Geometry: final body of the model. Coordinates: model frame, mm. A direction names the side the tool comes from. Give positions to 0.01 mm unless a question says otherwise; leave off trailing zeros. Order: outer loops, then holes, each group sorted by start corner. A loop starts at its lowest first (then second) coordinate and runs counter-clockwise, first axis right, second up. Notation, with made-up numbers: (27, 31.5) -> (38, 31.5) arc R24 ccw to (38, 55.5) -> close; hole circle Ø1 at (71, 35). An arc over 180 degrees is marked (long way). Write item = value, one per line.
Autodesk Inventor part; units mm, degrees
ref_plane "YZ Plane" through (0, 0, 0) normal (1, 0, 0) x (0, 1, 0)
ref_plane "XZ Plane" through (0, 0, 0) normal (0, 1, 0) x (-1, 0, 0)
ref_plane "XY Plane" through (0, 0, 0) normal (0, 0, 1) x (1, 0, 0)
sketch "Sketch1" plane through (0, 0, 0) normal (0, 0, 1) x (1, 0, 0)
  circle A0 centre (0, 0) radius 5.75
  circle A1 centre (0, 8) radius 2
  circle A2 centre (8, 0) radius 2
  circle A3 centre (0, -8) radius 2
  circle A4 centre (-8, 0) radius 2
  line L0 (-15, 17.5) -> (15, 17.5)
  line L1 (15, 17.5) -> (15, -17.5)
  line L2 (15, -17.5) -> (-15, -17.5)
  line L3 (-15, -17.5) -> (-15, 17.5)
  line L4 (-15, 17.5) -> (15, -17.5) construction
  line L5 (15, 17.5) -> (-15, -17.5) construction
  dimension "d0" = 11.5
  dimension "d2" = 4
  dimension "d3" = 4
  dimension "d4" = 4
  dimension "d5" = 4
  dimension "d6" = 30
  dimension "d7" = 35
extrude "Extrusion1" add sketch "Sketch1" along normal blind 25
sketch "Sketch2" plane through (-15, -17.5, 0) normal (0, -1, 0) x (1, 0, 0)
  line L0 (0, 0) -> (0, 25)
  line L1 (30, 0) -> (0, 0)
  line L2 (0, 25) -> (30, 0)
  line L3 (-15, 32.5) -> (45, 32.5)
  line L4 (45, 32.5) -> (45, -7.5)
  line L5 (45, -7.5) -> (-15, -7.5)
  line L6 (-15, -7.5) -> (-15, 32.5)
  line L7 (-15, 32.5) -> (45, -7.5) construction
  line L8 (45, 32.5) -> (-15, -7.5) construction
  point P0 (15, 0)
  point P1 (15, 12.5)
  dimension "d10" = 60
  dimension "d11" = 40
extrude "Extrusion2" add sketch "Sketch2" along normal blind 6 contours L0 L2 L1 | L3 L4 L5 L6
sketch "Sketch3" plane through (-15, -23.5, 0) normal (0, -1, 0) x (1, 0, 0)
  line L0 (-15, -7.5) -> (-15, 32.5)
  line L1 (45, 32.5) -> (45, -7.5)
  line L2 (-15, 26) -> (45, 26)
  line L3 (-15, 19) -> (45, 19)
  line L4 (-15, 6) -> (45, 6)
  line L5 (-15, -1) -> (45, -1)
  line L6 (45, 26) -> (45, 19)
  line L7 (45, 6) -> (45, -1)
  line L8 (-15, -1) -> (-15, 6)
  line L9 (-15, 19) -> (-15, 26)
  point P0 (15, 0)
extrude "Extrusion3" add sketch "Sketch3" along normal blind 1.5 contours L0 L4 L1 L5 | L0 L2 L1 L3
sketch "Sketch4" plane through (-15, -25, 0) normal (0, -1, 0) x (1, 0, 0)
  line L0 (-15, 26) -> (45, 26)
  line L1 (45, 26) -> (30, 19)
  line L2 (-15, 19) -> (45, 19)
  line L3 (30, 0) -> (30, 25)
  line L4 (30, 13) -> (5, 13)
  line L5 (5, 0) -> (5, 25)
  line L6 (45, -7.5) -> (-15, -7.5)
  line L7 (15, -7.5) -> (15, 32.5)
  line L8 (45, 32.5) -> (-15, 32.5)
  point P0 (15, 0)
  point P1 (37.5, 22.5)
  point P2 (37.5, 3.5)
  point P3 (-7.5, 22.5)
  point P4 (-7.5, 3.5)
hole "Hole1" at (22.5, -25, 22.5) at (22.5, -25, 3.5) at (-22.5, -25, 22.5) at (-22.5, -25, 3.5) direction (0, 1, 0) diameter 5.5 end through all counterbore diameter 10 counterbore depth 1.5
fillet "Fillet1" radius 2 8 edges at (15, 17.5, 12.5) (0, 17.5, 25) (-15, 17.5, 12.5) (0, 17.5, 0) (-30, -20.5, -7.5) (30, -20.5, -7.5) (30, -20.5, 32.5) (-30, -20.5, 32.5)
properties part number "CarroZ - EixoZ"
1) Section query C-C (x = 22.5). Output: boundary loops of the cut face in (y, z), plus the area to 3 significant figures.
Check sheet entries:
outline = (-23.5, -7.5) -> (-17.5, -7.5) -> (-17.5, 0.75) -> (-23.5, 0.75) -> close; (-23.5, 6.25) -> (-17.5, 6.25) -> (-17.5, 19.75) -> (-23.5, 19.75) -> close; (-23.5, 25.25) -> (-17.5, 25.25) -> (-17.5, 32.5) -> (-23.5, 32.5) -> close
area = 174 mm²
2) First-contact query: P1, Ø10, axis at x = 21.5, y = -16, coming from the +Z side; P2, Ø10, axis at x = -6, y = 3, coming from the -Z side; P3, Ø6.5, axis at x = 22.5, z = 3.5, coming from the -Y side; P4, Ø5, axis at x = 22.5, z = 22.5, coming from the -Y side. Flat tips, straight axial feed; report the tip coordinate or a pass-through.
Check sheet entries:
P1 = 32.5
P2 = 0
P3 = -23.5
P4 = through
3) Line query: line 1 (X direction, y = -19.1, z = 22.5); line 2 (Z direction, x = -22.5, y = -21.45); line 3 (Y direction, x = 0, z = 15.5). Output: solid intervals per line, ascending. Write a range as from..to.
Check sheet entries:
line_1 = -30..-25.25, -19.75..19.75, 25.25..30
line_2 = -7.5..0.75, 6.25..19.75, 25.25..32.5
line_3 = -23.5..-10, -6..-5.75, 5.75..6, 10..17.5
4) Mould query, pull axis Y, two halves, no side actions, for faces 1 (the face through (0, -24, 26)), 2 (the face through (6, 0, 12)), 3 (the face through (28, -25, 23)), 4 (the face through (14.43, 16.9, 12.68)). Classes: +Y half, -Y half, draft (parallel to the pull), parting line (faces both ways), or undercut.
Check sheet entries:
face_1 = draft
face_2 = undercut
face_3 = -Y half
face_4 = +Y half
5) Section query D-D (z = 12.5). Output: boundary loops of the cut face in (x, y), plus the area to 3 significant figures.
Check sheet entries:
outline = (-30, -23.5) -> (30, -23.5) -> (30, -17.5) -> (15, -17.5) -> (15, 15.5) arc R2 ccw to (13, 17.5) -> (-13, 17.5) arc R2 ccw to (-15, 15.5) -> (-15, -17.5) -> (-30, -17.5) -> close; hole circle Ø4 at (-8, 0); hole circle Ø11.5 at (0, 0); hole circle Ø4 at (0, -8); hole circle Ø4 at (0, 8); hole circle Ø4 at (8, 0)
area = 1,250 mm²
6) Section query B-B (y = -21.5). Output: boundary loops of the cut face in (x, z), plus the area to 3 significant figures.
Check sheet entries:
outline = (-30, -5.5) arc R2 ccw to (-28, -7.5) -> (28, -7.5) arc R2 ccw to (30, -5.5) -> (30, 30.5) arc R2 ccw to (28, 32.5) -> (-28, 32.5) arc R2 ccw to (-30, 30.5) -> close; hole circle Ø5.5 at (-22.5, 3.5); hole circle Ø5.5 at (-22.5, 22.5); hole circle Ø5.5 at (22.5, 3.5); hole circle Ø5.5 at (22.5, 22.5)
area = 2,300 mm²
7) Reachability of faces 5 (the face through (-29, -25, 3)), 6 (the face through (-15, -1, 12)), 7 (the face through (0, -24, -1)), 8 (the face through (17.738, -24.24, 1.977)), 9 (the face through (-28, -24, 19)) from +Z, -Z, +X, -X, +Y, -Y: full face, straight path, thin tool, end or side. Return the list, or none.
Check sheet entries:
face_5 = +Z, -Z, +X, -X, -Y
face_6 = +Z, -Z, -X, +Y
face_7 = -Z, +X, -X, -Y
face_8 = -Y
face_9 = +X, -X, -Y
8) Section query A-A (z = 3.5). Count the separate pieces of the cut face and the enclosed holes in it, plus the area to 3 significant figures.
Check sheet entries:
separate_pieces = 3
enclosed_holes = 5
area = 1,250 mm²
